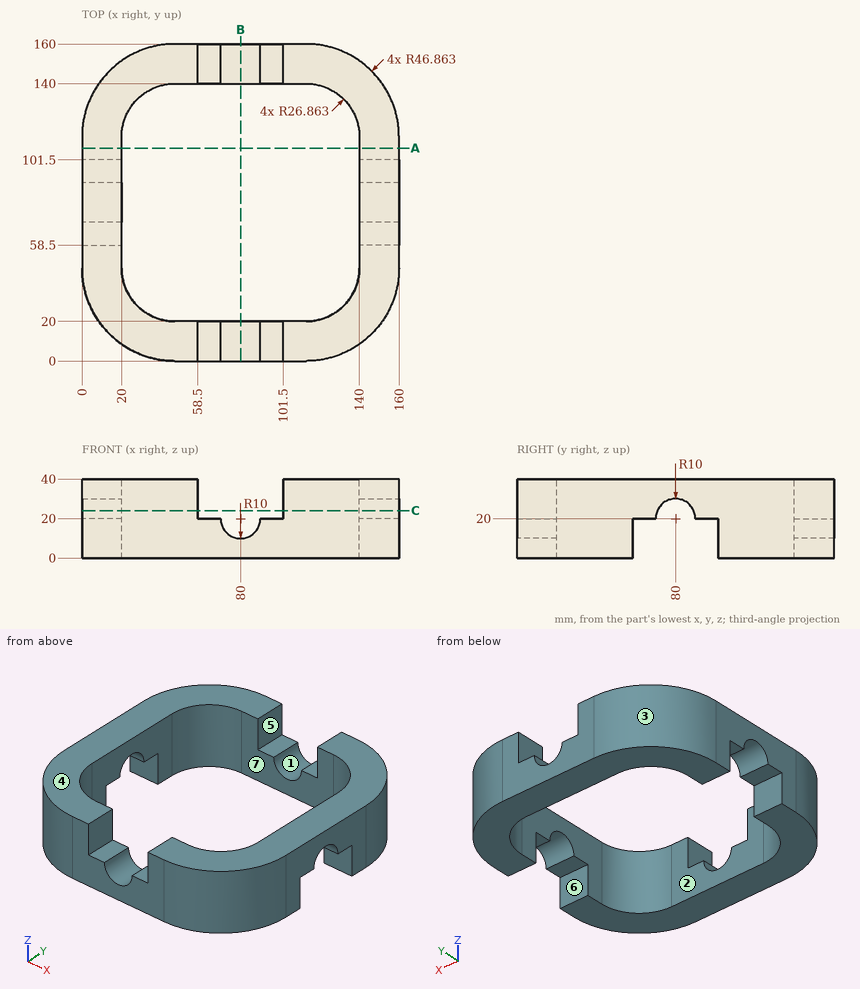
Source: three-view drawing plus pictorial views. Frame: mm from the lowest corner of the part. A direction names the side the tool comes from. Give positions to 0.01 mm unless a question says otherwise; leave off trailing zeros. Write each loop counter-clockwise with the first axis right and the second up, starting at its lowest first coordinate (ties: lowest second). Pieces come first, ordered by that corner, then holes. Notation, with made-up numbers: (34.25, -20.5) - (77.25, -20.5) arc R15 cw to (77.25, -14.5) - close; hole circle Ø2 at (14, 57.5). An arc over 180 degrees is marked (long way). Write item = value, one per line. Start each with the question number.
Q1. Cut plane C-C, the plane z = 24. Give the number of separate pieces and of enclosed holes in the cut face, then the cut area to 3 significant figures.
Q2. Material intervals for probe 1 along Y at (x, z) = (71, 2.5); probe 2 along X at (y, z) = (45.5, 34.5); probe 3 along X at (y, z) = (145, 12), sorted ascending.
Q3. Reachability of the marked faces 4, 5, 6 and 7 from +Z, -Z, +X, -X, +Y, -Y: full face, straight path, thin tool, end or side. Return the list, or none.
Q4. Pin query (flat end, axial travel): pin 1 Ø6 at (y, z) = (146.5, 31) entering from -X; pin 2 Ø6 at (y, z) = (151.5, 30.5) entering from +X; pin 3 Ø10 at (x, z) = (149.5, 11.5) entering from -Y. Return the tip coordinate at first contact, or that it passes through.
Q5. Cut plane B-B, the plane x = 80. Return loops of the section in (y, z).
Q6. Draft query along Y for the marked faces 1, 2 and 3. Return one class per face: +Y half, -Y half, draft (parallel to the pull), parting line (faces both ways), or undercut.
Q7. Cut plane A-A, the plane y = 107.5. Return loops of the section in (x, z), then the cut area to 3 significant figures.
Computed values:
q1.separate_pieces = 4
q1.enclosed_holes = 0
q1.area = 7,480 mm²
q2.probe_1 = 0 to 20, 140 to 160
q2.probe_2 = 0.02 to 20.03, 139.97 to 159.98
q2.probe_3 = 12.5 to 74, 86 to 147.5
q3.face_4 = +Z, +X, -X, +Y, -Y
q3.face_5 = +Z, +Y, -Y
q3.face_6 = -Z, +X, -X
q3.face_7 = +Z, -Z
q4.pin_1 = 11.17
q4.pin_2 = 143.89
q4.pin_3 = 12.04
q5.outline = (0, 0) - (20, 0) - (20, 10) - (0, 10) - close; (140, 0) - (160, 0) - (160, 10) - (140, 10) - close
q6.face_1 = draft
q6.face_2 = undercut
q6.face_3 = +Y half
q7.outline = (0, 0) - (20, 0) - (20, 40) - (0, 40) - close; (140, 0) - (160, 0) - (160, 40) - (140, 40) - close
q7.area = 1,600 mm²
